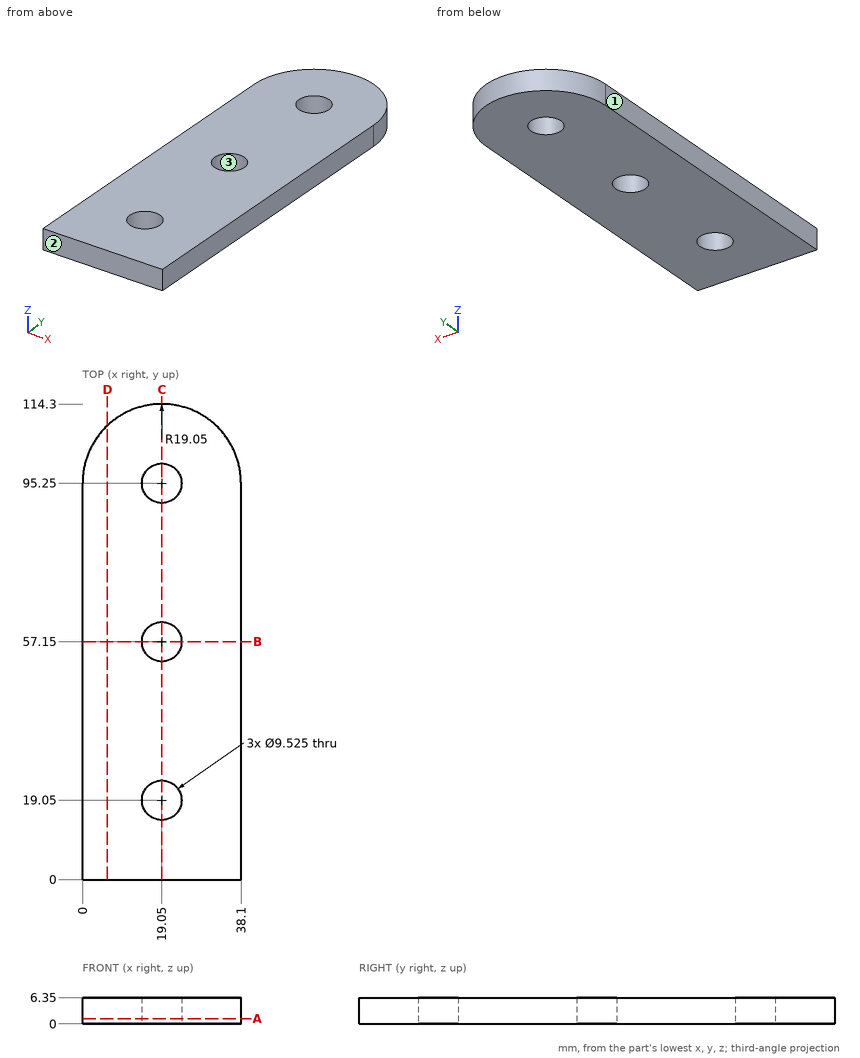
Geometry check sheet. Reference: drawing and pictorial views, mm from the part's lowest x, y, z. Give positions to 0.01 mm unless a question says otherwise; leave off trailing zeros. Loops run counter-clockwise (first coordinate to the right, second up) from the corner with the lowest first, then second, coordinate; pieces in that order, holes last. Notation, with made-up numbers: (4, 80) -> (15, 80) arc R11 ccw to (15, 88) -> close; hole circle Ø6 at (-10.5, 48.5). An arc over 180 degrees is marked (long way). Answer in a Markdown table with one row per item. Add a question column.
1) Material ranges on probe 1 along Y at (x, z) = (19.05, 1.75); probe 2 along X at (y, z) = (108, 2); probe 3 along Y at (x, z) = (35.5, 1.5), recorded low to high. Write a range as from..to.
2) Cross-section at D-D on x = 6. Record the boundary of the cut face in (y, z), and give its area (3 significant figures).
3) Cross-section at A-A on z = 1.25. State how many separate pieces and enclosed holes the cut face has, and give its area (3 significant figures).
4) Cross-section at C-C on x = 19.05. Record the boundary of the cut face in (y, z), and give its area (3 significant figures).
5) Gauge pin test, flat ends, axial feed: P1, Ø10, axis at x = 23.5, y = 94, coming from the -Z side; P2, Ø2, axis at x = 17.5, z = 5.5, coming from the +Y side. Record the tip position at first contact, or that the pin passes through.
6) Cross-section at B-B on y = 57.15. Record the boundary of the cut face in (x, z).
7) Draft check along Y on the marked faces 1, 2 and 3. Enter one of: pulls with the +Y half, pulls with the -Y half, needs draft (parallel to the pull), parting line crosses it, or undercut.
Outcome:
| question | item | result |
|---|---|---|
| 1 | probe 1 | y = 0..14.29, 23.81..52.39, 61.91..90.49, 100.01..114.3 |
| 1 | probe 2 | x = 4.9..33.2 |
| 1 | probe 3 | y = 0..104.86 |
| 2 | outline | (0, 0) -> (109.13, 0) -> (109.13, 6.35) -> (0, 6.35) -> close |
| 2 | area | 693 mm^2 |
| 3 | separate pieces | 1 |
| 3 | enclosed holes | 3 |
| 3 | area | 3,990 mm^2 |
| 4 | outline | (0, 0) -> (14.29, 0) -> (14.29, 6.35) -> (0, 6.35) -> close; (23.81, 0) -> (52.39, 0) -> (52.39, 6.35) -> (23.81, 6.35) -> close; (61.91, 0) -> (90.49, 0) -> (90.49, 6.35) -> (61.91, 6.35) -> close; (100.01, 0) -> (114.3, 0) -> (114.3, 6.35) -> (100.01, 6.35) -> close |
| 4 | area | 544 mm^2 |
| 5 | P1 | stops at z = 0 |
| 5 | P2 | stops at y = 114.29 |
| 6 | outline | (0, 0) -> (14.29, 0) -> (14.29, 6.35) -> (0, 6.35) -> close; (23.81, 0) -> (38.1, 0) -> (38.1, 6.35) -> (23.81, 6.35) -> close |
| 7 | face 1 | needs draft |
| 7 | face 2 | pulls with the -Y half |
| 7 | face 3 | undercut |
